from build123d import *

# Parameters (mm, degrees)
SKETCH4_W           = 20
SKETCH4_H           = 20
BOSS_EXTRUDE2_DEPTH = 200
SKETCH5_R           = 2.5
BOSS_EXTRUDE3_DEPTH = 3


with BuildPart() as part:
    # Sketch4 → Boss-Extrude2 (new body)
    with BuildSketch(Plane(origin=(0, 0, 0), x_dir=(1, 0, 0), z_dir=(0, 1, 0))):
        with Locations((10, -10)):
            Rectangle(SKETCH4_W, SKETCH4_H)
    extrude(amount=BOSS_EXTRUDE2_DEPTH)

    # Sketch5 → Boss-Extrude3 (add)
    with BuildSketch(Plane.XY.offset(20)):
        with Locations(Location((10, 150, 0), (0, 0, 180))):
            Circle(SKETCH5_R)
        with Locations(Location((10, 130, 0), (0, 0, 180))):
            Circle(SKETCH5_R)
    extrude(amount=BOSS_EXTRUDE3_DEPTH)


solid = part.part
The model under review builds one solid part; all positions refer to its coordinate system, in mm. A direction names the side the tool comes from. Give positions to 0.01 mm unless a question says otherwise; leave off trailing zeros. Order: outer loops, then holes, each group sorted by start corner. A loop starts at its lowest first (then second) coordinate and runs counter-clockwise, first axis right, second up. Notation, with made-up numbers: M -7,10.5 L 45,10.5 A26 cw 45,41.5 Z; hole C 35,16.5 d5. An arc over 180 degrees is marked long. Answer in a Markdown table with one row per item. Add a question column.
1. Machinability: for faces 4 (the flat face through (10, 130, 23)), 5 (the cylindrical face through (10.33, 127.52, 21.48)), which of the approach directions +Z, -Z, +X, -X, +Y, -Y give a long, thin tool a straight path to every point of the face, cutting with its end or side? Answer none if there is none.
2. Add section A-A on x = 10. State the section outline as (y, z) points, plus the area to 3 significant figures.
3. Add section C-C on x = 18. State the section outline as (y, z) points.
4. To check wall thickness, follow line 1 along Z through (x, y) = (12.25, 101). State the ranges of the line that lie inside material, in increasing order.
5. For pin 1 Ø3 at (x, y) = (17.5, 35) entering from +Z, flat-tipped, find the tip position at first contact; note if it passes through.
6. Add section B-B on y = 150. State the section outline as (x, z) points, plus the area to 3 significant figures.
7. Mouldability with a two-part tool opening along Y and no side actions: class faces 1 (the flat face through (10, 0, 10)), 2 (the flat face through (10, 150, 23)), 3 (the cylindrical face through (10.33, 147.52, 21.48)) as released by +Y, released by -Y, zero draft, split by the parting line, or undercut.
8. Add section D-D on y = 174. State the section outline as (x, z) points, plus the area to 3 significant figures.
The answers:
| question | item | result |
|---|---|---|
| 1 | face 4 | +Z, +X, -X, +Y, -Y |
| 1 | face 5 | +Z |
| 2 | outline | M 0,0 L 200,0 L 200,20 L 152.5,20 L 152.5,23 L 147.5,23 L 147.5,20 L 132.5,20 L 132.5,23 L 127.5,23 L 127.5,20 L 0,20 Z |
| 2 | area | 4,030 mm2 |
| 3 | outline | M 0,0 L 200,0 L 200,20 L 0,20 Z |
| 4 | line 1 | 0 to 20 |
| 5 | pin 1 | z = 20 |
| 6 | outline | M 0,0 L 20,0 L 20,20 L 12.5,20 L 12.5,23 L 7.5,23 L 7.5,20 L 0,20 Z |
| 6 | area | 415 mm2 |
| 7 | face 1 | released by -Y |
| 7 | face 2 | zero draft |
| 7 | face 3 | undercut |
| 8 | outline | M 0,0 L 20,0 L 20,20 L 0,20 Z |
| 8 | area | 400 mm2 |
